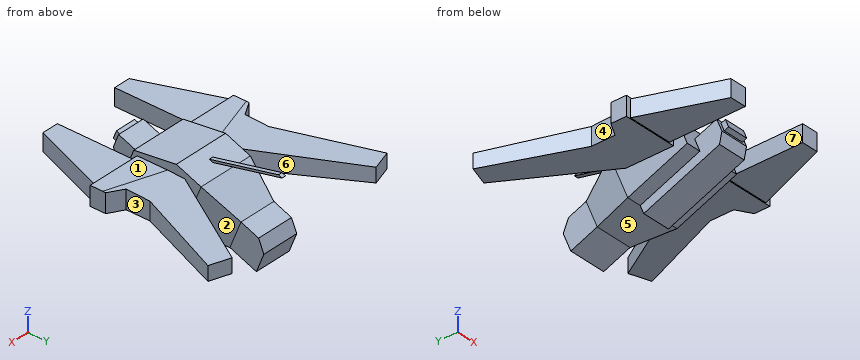
```python
from build123d import *
from OCP.BRepFilletAPI import BRepFilletAPI_MakeChamfer

# Parameters (mm, degrees)
BOSS_EXTRUDE1_DEPTH  = 5.08
CHAMFER5_SIZE        = 1.27
CHAMFER5_SIZE2       = 33.019999999999996
SKETCH6_W            = 12.052934308980802
SKETCH6_H            = 4.563994413231876
BOSS_EXTRUDE2_DEPTH  = 20.32
CHAMFER6_SIZE        = 20.32
CHAMFER6_SIZE_2      = 7.62
BOSS_EXTRUDE5_DEPTH  = 19.05
CUT_EXTRUDE4_DEPTH   = 15.494
CUT_EXTRUDE5_DEPTH   = 15.494
CUT_EXTRUDE6_DEPTH   = 15.494
CUT_EXTRUDE7_DEPTH   = 15.494
CHAMFER7_SIZE        = 25.4
CHAMFER7_SIZE_2      = 13.97
CUT_EXTRUDE9_DEPTH   = 15.494
BOSS_EXTRUDE7_DEPTH  = 6.35
SKETCH24_W           = 3.7386650704626128
SKETCH24_H           = 3.778783012789209
SKETCH24_W_2         = 3.9045544155871448
SKETCH24_H_2         = 3.7787830127892117
CUT_EXTRUDE11_DEPTH  = 19.05
CHAMFER9_SIZE        = 2.54
CHAMFER9_SIZE2       = 3.8099999999999996
SKETCH26_W           = 23.370745721099873
SKETCH26_H           = 31.500943766528344
CUT_EXTRUDE14_DEPTH  = 1.2699999999999978
SKETCH27_W           = 5.63305406156012
SKETCH27_H           = 2.3288196199824216
BOSS_EXTRUDE9_DEPTH  = 1.2699999999999978
SKETCH30_W           = 1.0845533410304151
SKETCH30_H           = 1.0329414918412994
SKETCH34_W           = 15.244980385835458
SKETCH34_H           = 13.062490152383763
BOSS_EXTRUDE14_DEPTH = 10.16
CHAMFER11_SIZE       = 2.54
CHAMFER11_SIZE_2     = 10.16
SKETCH38_W           = 10.164980385835456
SKETCH38_H           = 7.9824901523837575
BOSS_EXTRUDE15_DEPTH = 7.62
CHAMFER12_SIZE       = 2.54


# Some blends are built 0.0001 mm under size
with BuildPart() as part:
    # Sketch4 → Boss-Extrude1 (new body)
    with BuildSketch(Plane.XY):
        Polygon((0, 0), (0, 12.7), (-14.664448494293428, 38.099999999999994), (-20.084228903343057, 36.328898401943476), (-10.761091691630092, 12.71368779454834), (-10.761091691630092, 6.3636877945483405), (-14.57109169163009, 4.164020520404326), (-14.57109169163009, 0), align=None)
    extrude(amount=BOSS_EXTRUDE1_DEPTH)

    # Chamfer5
    chamfer5_edges = [part.edges().sort_by_distance(p)[0] for p in [
        (-17.374338698818242, 37.214449200971735, 5.08),
    ]]
    chamfer5_side = [part.faces().sort_by_distance(p)[0] for p in [
        (-17.374338698818242, 37.214449200971735, 2.54),
    ]]
    chamfer(chamfer5_edges, length=CHAMFER5_SIZE, length2=CHAMFER5_SIZE2, reference=chamfer5_side[0])

    # Sketch6 → Boss-Extrude2 (add)
    with BuildSketch(Plane.XZ):
        with Locations((-7.2855458458150455, 2.54)):
            Rectangle(SKETCH6_W, SKETCH6_H)
    extrude(amount=BOSS_EXTRUDE2_DEPTH)

    # Chamfer6
    # the kernel refuses this chamfer: 20.32, 7.62 mm, written as the material it takes off along each edge
    with BuildSketch(Plane(origin=(-13.312013000305447, -20.32, 57.52944740394708), x_dir=(-0.013536660009854505, 0.9999083752203387, 0), z_dir=(0, 0, -1))) as chamfer6_piece_1_section:
        Polygon((CHAMFER6_SIZE * 0.99990837522, CHAMFER6_SIZE * 0.0135366600099), (-CHAMFER6_SIZE_2 * 0.0135366600099, CHAMFER6_SIZE_2 * 0.99990837522), (0, 0), align=None)
    chamfer6_piece_1 = extrude(amount=109.97889480789416, mode=Mode.PRIVATE)
    chamfer6_piece_1 = split(chamfer6_piece_1, bisect_by=Plane(origin=(-10.948471131308636, 0, 2.5400000000000014), z_dir=(0, -1, 0)), keep=Keep.TOP, mode=Mode.PRIVATE)
    add(chamfer6_piece_1, mode=Mode.SUBTRACT)


with BuildPart() as body_2:
    # Mirror8: mirrored copy
    add(part.part.mirror(Plane(origin=(7.619999999999999, 0, 0), x_dir=(0, 0, 1), z_dir=(1, 0, 0))))


with BuildPart() as part_1:
    add(part.part)

    add(body_2.part)  # Boss-Extrude5 merges body 2
    # Sketch7 → Boss-Extrude5 (add, symmetric)
    with BuildSketch(Plane(origin=(0, 0, 0), x_dir=(0, -1, 0), z_dir=(0, 0, 1))):
        Polygon((5.0986751933069705, 0), (5.0986751933069705, 15.280255393277036), (-20.245687537827482, 15.239999999999998), (-20.245687537827482, 0), align=None)
    extrude(amount=BOSS_EXTRUDE5_DEPTH, both=True)

    # Sketch13 → Cut-Extrude4 (cut)
    with BuildSketch(Plane(origin=(15.272118449240836, 0.02425727333804481, 0), x_dir=(0, 0, -1), z_dir=(0.9999987385949102, 0.0015883351625656467, 0))):
        Polygon((-19.05, 4.286246257710902), (4.496404811954787, -5.122938928746256), (-19.05, -5.122938928746256), align=None)
    extrude(amount=-CUT_EXTRUDE4_DEPTH, mode=Mode.SUBTRACT)

    # Sketch18 → Cut-Extrude5 (cut)
    with BuildSketch(Plane(origin=(0, -5.0986751933069705, 19.05), x_dir=(0, 0, -1), z_dir=(1, 0, 0))):
        Polygon((38.1, 0), (38.1, 25.344362731134453), (33.61333406805571, 25.344362731134453), (23.485668928436706, 0), align=None)
    extrude(amount=CUT_EXTRUDE5_DEPTH, mode=Mode.SUBTRACT)

    # Sketch19 → Cut-Extrude6 (cut)
    with BuildSketch(Plane.ZY):
        Polygon((12.672573032991338, 20.245687537827482), (19.05, 4.286251664410568), (19.05, 20.245687537827482), align=None)
    extrude(amount=-CUT_EXTRUDE6_DEPTH, mode=Mode.SUBTRACT)

    # Sketch20 → Cut-Extrude7 (cut)
    with BuildSketch(Plane.ZY):
        Polygon((-10.813095895445443, 10.860760680109815), (12.672573032991338, 20.245687537827482), (-14.563334068055712, 20.245687537827482), align=None)
    extrude(amount=-CUT_EXTRUDE7_DEPTH, mode=Mode.SUBTRACT)

    # Chamfer7
    # the kernel refuses this chamfer: 25.4, 13.97 mm, written as the material it takes off along each edge
    with BuildSketch(Plane(origin=(-65.73691449265259, 4.196216304667381, 19.08597833505926), x_dir=(-0.0014746788980924302, 0.9353516299299037, -0.3537162050424322), z_dir=(0.9999989122833349, 0.0013696301766686866, -0.0005473073417378643))) as chamfer7_piece_1:
        Polygon((CHAMFER7_SIZE * 0.999826618339, -CHAMFER7_SIZE * 0.018620774985), (-CHAMFER7_SIZE_2 * 0.018620774985, -CHAMFER7_SIZE_2 * 0.999826618339), (0, 0), align=None)
    extrude(amount=146.73930435250884, mode=Mode.SUBTRACT)

    # Sketch21 → Cut-Extrude9 (cut)
    with BuildSketch(Plane.ZY):
        Polygon((8.477655483236292, 18.569388919356417), (4.825777553004942, 17.110090171129713), (7.479050890335823, 10.47030489395858), align=None)
    extrude(amount=-CUT_EXTRUDE9_DEPTH, mode=Mode.SUBTRACT)

    # Sketch22 → Boss-Extrude7 (add)
    with BuildSketch(Plane(origin=(0.00455562028050382, -2.868169540906279, 1.1461270887773878), x_dir=(0.9999989122833348, 0.0013696301766686846, -0.0005473073417378687), z_dir=(0.001474934624707707, -0.9286029793832664, 0.3710718680368721))):
        Polygon((7.635563761108569, -6.010956849215719), (11.537018076990257, -6.010956849215718), (11.537018076990257, 1.5466091763627066), (3.899998790351411, 1.5466091763627066), (3.899998790351413, -6.010956849215722), align=None)
    extrude(amount=BOSS_EXTRUDE7_DEPTH)

    # Sketch24 → Cut-Extrude11 (cut)
    with BuildSketch(Plane(origin=(0.00455562028050382, -2.868169540906279, 1.1461270887773878), x_dir=(0.9999989122833348, 0.0013696301766686846, -0.0005473073417378687), z_dir=(0.001474934624707707, -0.9286029793832664, 0.3710718680368722))):
        with Locations((13.406350612221562, -4.121565342821113)):
            Rectangle(SKETCH24_W, SKETCH24_H)
        with Locations((1.9477215825578391, -4.121565342821115)):
            Rectangle(SKETCH24_W_2, SKETCH24_H_2)
    extrude(amount=-CUT_EXTRUDE11_DEPTH, mode=Mode.SUBTRACT)

    # Chamfer9
    chamfer9_edges = [part_1.edges().sort_by_distance(p)[0] for p in [
        (7.73242149326798, -10.984726370799283, -2.083589456062718),
    ]]
    chamfer9_side = [part_1.faces().sort_by_distance(p)[0] for p in [
        (7.714767768751576, -0.06198305402502739, -6.44834259236495),
    ]]
    chamfer(chamfer9_edges, length=CHAMFER9_SIZE, length2=CHAMFER9_SIZE2, reference=chamfer9_side[0])

    # Sketch26 → Cut-Extrude14 (cut)
    with BuildSketch(Plane(origin=(0, -2.23049941287892, -5.581798510541238), x_dir=(-1, 0, 0), z_dir=(0, -0.37107227165836976, -0.9286039894412996))):
        with Locations((-7.42917145975186, 4.586757393504559)):
            Rectangle(SKETCH26_W, SKETCH26_H)
    extrude(amount=-CUT_EXTRUDE14_DEPTH, mode=Mode.SUBTRACT)

    # Sketch27 → Boss-Extrude9 (add)
    with BuildSketch(Plane(origin=(0.01392145514739876, -8.76479845999002, 3.5024334508115262), x_dir=(0.9999989122833348, 0.0013696301766687824, -0.0005473073417379074), z_dir=(0.0014749346247078124, -0.9286029793832665, 0.371071868036872))):
        with Locations((7.7185084336708325, -0.353981031334653)):
            Rectangle(SKETCH27_W, SKETCH27_H)
    extrude(amount=BOSS_EXTRUDE9_DEPTH)

    # Sweep3: sweep along a path in Sketch31
    with BuildLine(Plane(origin=(7.619999999999999, -5.0986751933069705, 19.05), x_dir=(0, 0, -1), z_dir=(1, 0, 0))) as sweep3_path:
        Line((12.859063600877302, 18.79247143047996), (8.75450408234446, 37.3194963828567))
    # Sketch30 → Sweep3 (sweep)
    with BuildSketch(Plane(origin=(0, 4.018830078140977, 10.057074937909151), x_dir=(1, 0, 0), z_dir=(0, 0.3710722716583693, 0.9286039894412997))):
        with Locations((7.6507653900392825, 10.410250498608775)):
            Rectangle(SKETCH30_W, SKETCH30_H)
    sweep(path=sweep3_path.line)

    # Sketch34 → Boss-Extrude14 (add)
    with BuildSketch(Plane(origin=(0, 13.091260092988732, -5.231297384904211), x_dir=(1, 0, 0), z_dir=(0, 0.9286039894412996, -0.3710722716583697))):
        with Locations((7.622490192917729, -4.299071239765427)):
            Rectangle(SKETCH34_W, SKETCH34_H)
    extrude(amount=BOSS_EXTRUDE14_DEPTH)

    # Chamfer11
    chamfer11_edges_1 = [part_1.edges().sort_by_distance(p)[0] for p in [
        (15.244980385835458, 24.121142756673255, -5.009256960814719),
    ]]
    chamfer11_side_1 = [part_1.faces().sort_by_distance(p)[0] for p in [
        (15.194180385835457, 24.121142756673255, -5.009256960814719),
    ]]
    chamfer11_edges_2 = [part_1.edges().sort_by_distance(p)[0] for p in [
        (7.622490192917729, 21.697578809493194, -11.074197194585345),
    ]]
    chamfer11_side_2 = [part_1.faces().sort_by_distance(p)[0] for p in [
        (7.622490192917729, 21.650405726829575, -11.0553467231851),
    ]]
    chamfer11_edges_3 = [part_1.edges().sort_by_distance(p)[0] for p in [
        (0, 24.121142756673255, -5.009256960814719),
    ]]
    chamfer11_side_3 = [part_1.faces().sort_by_distance(p)[0] for p in [
        (0, 24.073969674009636, -4.9904064894144735),
    ]]
    chamfer11_edges_4 = [part_1.edges().sort_by_distance(p)[0] for p in [
        (7.622490192917729, 26.54470670385332, 1.055683272955907),
    ]]
    chamfer11_side_4 = [part_1.faces().sort_by_distance(p)[0] for p in [
        (7.622490192917729, 26.4975336211897, 1.074533744356152),
    ]]
    chamfer11 = BRepFilletAPI_MakeChamfer(part_1.part.solid().wrapped)
    for e in chamfer11_edges_1:
        chamfer11.Add(CHAMFER11_SIZE - 0.0001, CHAMFER11_SIZE_2 - 0.0001, e.wrapped, chamfer11_side_1[0].wrapped)
    for e in chamfer11_edges_2:
        chamfer11.Add(CHAMFER11_SIZE_2 - 0.0001, CHAMFER11_SIZE - 0.0001, e.wrapped, chamfer11_side_2[0].wrapped)
    for e in chamfer11_edges_3:
        chamfer11.Add(CHAMFER11_SIZE_2 - 0.0001, CHAMFER11_SIZE - 0.0001, e.wrapped, chamfer11_side_3[0].wrapped)
    for e in chamfer11_edges_4:
        chamfer11.Add(CHAMFER11_SIZE_2 - 0.0001, CHAMFER11_SIZE - 0.0001, e.wrapped, chamfer11_side_4[0].wrapped)
    add(Compound.cast(chamfer11.Shape()), mode=Mode.REPLACE)  # a hair under: the kernel refuses the full size

    # Sketch38 → Boss-Extrude15 (add)
    with BuildSketch(Plane(origin=(0, 22.525876625712346, -9.001391664953251), x_dir=(1, 0, 0), z_dir=(0, 0.9286039894412996, -0.37107227165836976))):
        with Locations((7.622490192917729, -4.299071239765427)):
            Rectangle(SKETCH38_W, SKETCH38_H)
    extrude(amount=BOSS_EXTRUDE15_DEPTH)

    # Chamfer12
    chamfer12_edges = [part_1.edges().sort_by_distance(p)[0] for p in [
        (7.622490192917728, 32.67814553338378, -4.130541570261777),
    ]]
    chamfer(chamfer12_edges, length=CHAMFER12_SIZE)


solid = part_1.part
```
Can you work these out from the model? Positions are in its coordinate system, mm. Face numbers are marked on the shaded views. A direction names the side the tool comes from. Give positions to 0.01 mm unless a question says otherwise; leave off trailing zeros. Loops run counter-clockwise (first coordinate to the right, second up) from the corner with the lowest first, then second, coordinate; pieces in that order, holes last. Notation, with made-up numbers: M -2,-20 L 57,-20 A16 cw 57,8 Z; hole C 78.5,34 d6. An arc over 180 degrees is marked long. One line per item, written item: value.
(1) I need wall thicknesses on line 1 (X direction, y = 7, z = 3.5); line 2 (X direction, y = 6.5, z = -6.25); line 3 (Z direction, x = -6, y = 6). Which ranges of each line are inside material? Lowest first, please.
Returned:
line 1: -10.76 to 26
line 2: 3.89 to 11.52
line 3: 0 to 5.08
(2) We'd pull the mould along X, two halves only. Please class the marked faces 4, 5, 6 and 7: released by +X, released by -X, zero draft, split by the parting line, or undercut.
Returned:
face 4: released by -X
face 5: zero draft
face 6: undercut
face 7: undercut
(3) Suppose I cut it at B-B on y = 27. List the corners of the cut face in (x, z) for me.
Returned:
outline: M -16.4,0 L -8.26,0 L -8.26,4.29 L -16.4,4.2 Z; M 2.54,-10.46 L 12.7,-10.46 L 12.7,-1.86 L 2.54,-1.86 Z; M 7.11,8.85 L 8.19,8.85 L 8.19,9.44 L 7.11,9.44 Z; M 23.5,0 L 31.64,0 L 31.64,4.2 L 23.5,4.29 Z
(4) Suppose I cut it at D-D on x = -8. List the corners of the cut face in (y, z) for me, plus the area to 3 significant figures.
Returned:
outline: M -14.17,0.26 L 0,0.26 L 0,0 L 26.56,0 L 26.56,4.31 L 5.54,5.08 L 0,5.08 L 0,4.82 L -14.17,4.82 Z
area: 191 mm^2
(5) Suppose I cut it at A-A on y = -15.5. List the corners of the cut face in (x, z) for me, plus the area to 3 significant figures.
Returned:
outline: M -7.5,0.26 L -1.26,0.26 L -1.26,4.82 L -7.5,4.82 Z; M 16.5,0.26 L 22.74,0.26 L 22.74,4.82 L 16.5,4.82 Z
area: 57.0 mm^2
(6) Will these pins go through, and if not, where does the flat tip stop? pin 1 (10 mm diameter, centred on y = 19.5, z = 1.5, fed in from +X); pin 2 (1.5 mm diameter, centred on y = -3, z = 1.5, fed in from +X); pin 3 (9.5 mm diameter, centred on x = -10, y = -12.5, fed in from +Z).
Returned:
pin 1: x = 30.65
pin 2: x = 27.71
pin 3: z = 4.82
(7) Which directions (+Z, -Z, +X, -X, +Y, -Y) give clear straight access to the entire face, cutting with the end or side of a thin tool? Please do the marked faces 1, 2 and 3.
Returned:
face 1: +Z, +X, +Y, -Y
face 2: -Z, +Y
face 3: +Z, -Z, +X
